from build123d import *

# Parameters (mm, degrees)
SKETCH1_R           = 92.075
BOSS_EXTRUDE3_DEPTH = 92.075
SKETCH3_R           = 82.55
CUT_EXTRUDE1_DEPTH  = 82.55
FILLET12_R          = 82.55
FILLET13_R          = 92.075
SKETCH6_R           = 3.937
CUT_EXTRUDE3_DEPTH  = 50.8
SKETCH8_R           = 3.937
SKETCH8_R_2         = 1.4224
BOSS_EXTRUDE6_DEPTH = 3.175


with BuildPart() as part:
    # Sketch1 → Boss-Extrude3 (new body)
    with BuildSketch(Plane(origin=(0, 0, 0), x_dir=(1, 0, 0), z_dir=(0, 1, 0))):
        with Locations(Location((0, 0, 0), (0, 0, 270))):
            Circle(SKETCH1_R)
    extrude(amount=BOSS_EXTRUDE3_DEPTH)

    # Sketch3 → Cut-Extrude1 (cut)
    with BuildSketch(Plane(origin=(0, 92.075, 0), x_dir=(1, 0, 0), z_dir=(0, 1, 0))):
        with Locations(Location((0, 0, 0), (0, 0, 270))):
            Circle(SKETCH3_R)
    extrude(amount=-CUT_EXTRUDE1_DEPTH, mode=Mode.SUBTRACT)

    # Fillet12
    fillet12_edges = [part.edges().sort_by_distance(p)[0] for p in [
        (0, 9.525, -82.55),
    ]]
    fillet(fillet12_edges, radius=FILLET12_R - 0.0001)  # a hair under: the kernel refuses the full size

    # Fillet13
    fillet13_edges = [part.edges().sort_by_distance(p)[0] for p in [
        (0, 0, -92.075),
    ]]
    fillet(fillet13_edges, radius=FILLET13_R - 0.0001)  # a hair under: the kernel refuses the full size

    # Sketch6 → Cut-Extrude3 (cut)
    with BuildSketch(Plane(origin=(0, 92.075, 0), x_dir=(1, 0, 0), z_dir=(0, 1, 0))):
        with Locations(Location((0, 87.122, 0), (0, 0, 270))):
            Circle(SKETCH6_R)
        with Locations(Location((75.449865229, 43.561, 0), (0, 0, 270))):
            Circle(SKETCH6_R)
        with Locations(Location((75.449865229, -43.561, 0), (0, 0, 270))):
            Circle(SKETCH6_R)
        with Locations(Location((0, -87.122, 0), (0, 0, 270))):
            Circle(SKETCH6_R)
        with Locations(Location((-75.449865229, -43.561, 0), (0, 0, 270))):
            Circle(SKETCH6_R)
        with Locations(Location((-75.449865229, 43.561, 0), (0, 0, 270))):
            Circle(SKETCH6_R)
    extrude(amount=-CUT_EXTRUDE3_DEPTH, mode=Mode.SUBTRACT)

    # Sketch8 → Boss-Extrude6 (add)
    # profile 1 of 6: a face of its own
    with BuildSketch(Plane(origin=(0, 92.075, 0), x_dir=(1, 0, 0), z_dir=(0, 1, 0))):
        with Locations(Location((-75.449865229, -43.561, 0), (0, 0, 270))):
            Circle(SKETCH8_R)
        with Locations(Location((-75.449865229, -43.561, 0), (0, 0, 270))):
            Circle(SKETCH8_R_2, mode=Mode.SUBTRACT)
    # profile 2 of 6: a face of its own
    with BuildSketch(Plane(origin=(0, 92.075, 0), x_dir=(1, 0, 0), z_dir=(0, 1, 0))):
        with Locations(Location((0, -87.122, 0), (0, 0, 270))):
            Circle(SKETCH8_R)
        with Locations(Location((0, -87.122, 0), (0, 0, 270))):
            Circle(SKETCH8_R_2, mode=Mode.SUBTRACT)
    # profile 3 of 6: a face of its own
    with BuildSketch(Plane(origin=(0, 92.075, 0), x_dir=(1, 0, 0), z_dir=(0, 1, 0))):
        with Locations(Location((75.449865229, -43.561, 0), (0, 0, 270))):
            Circle(SKETCH8_R)
        with Locations(Location((75.449865229, -43.561, 0), (0, 0, 270))):
            Circle(SKETCH8_R_2, mode=Mode.SUBTRACT)
    # profile 4 of 6: a face of its own
    with BuildSketch(Plane(origin=(0, 92.075, 0), x_dir=(1, 0, 0), z_dir=(0, 1, 0))):
        with Locations(Location((75.449865229, 43.561, 0), (0, 0, 270))):
            Circle(SKETCH8_R)
        with Locations(Location((75.449865229, 43.561, 0), (0, 0, 270))):
            Circle(SKETCH8_R_2, mode=Mode.SUBTRACT)
    # profile 5 of 6: a face of its own
    with BuildSketch(Plane(origin=(0, 92.075, 0), x_dir=(1, 0, 0), z_dir=(0, 1, 0))):
        with Locations(Location((0, 87.122, 0), (0, 0, 270))):
            Circle(SKETCH8_R)
        with Locations(Location((0, 87.122, 0), (0, 0, 270))):
            Circle(SKETCH8_R_2, mode=Mode.SUBTRACT)
    # profile 6 of 6: a face of its own
    with BuildSketch(Plane(origin=(0, 92.075, 0), x_dir=(1, 0, 0), z_dir=(0, 1, 0))):
        with Locations(Location((-75.449865229, 43.561, 0), (0, 0, 270))):
            Circle(SKETCH8_R)
        with Locations(Location((-75.449865229, 43.561, 0), (0, 0, 270))):
            Circle(SKETCH8_R_2, mode=Mode.SUBTRACT)
    extrude(amount=-BOSS_EXTRUDE6_DEPTH)


solid = part.part
Work out the finished part from the listing and answer in its coordinate system (mm). Give positions to 0.01 mm unless a question says otherwise; leave off trailing zeros.
Q1. Given pin 1 (4 mm diameter, centred on x = -0.5, z = 87, fed in from -Y); pin 2 (12.5 mm diameter, centred on x = 75.45, z = 43.56, fed in from -Y); pin 3 (1.5 mm diameter, centred on x = 65.5, z = -28, fed in from +Y), each flat-ended and moving along its own axis, determine where each tip first touches the part or whether it passes through.
Answer:
pin 1: stops at y = 88.9
pin 2: stops at y = 48.06
pin 3: stops at y = 51.67
Q2. For a pull along Z with two mould halves and no side action, classify faces 1 (the face through (-1.508, 75.038, -83.485)), 2 (the face through (-47, 92.075, -69)), 3 (the face through (0.17, 75.04, 83.19)) as released by +Z, released by -Z, zero draft, split by the parting line, or undercut.
Answer:
face 1: undercut
face 2: zero draft
face 3: undercut
Q3. A straight line is drawn through the part: L1, parallel to Z at x = 0, y = 62 (3 decimals). Find the intervals that lie inside material, in ascending order.
Answer:
L1: z = -83.185 to -76.877, 76.877 to 83.185
